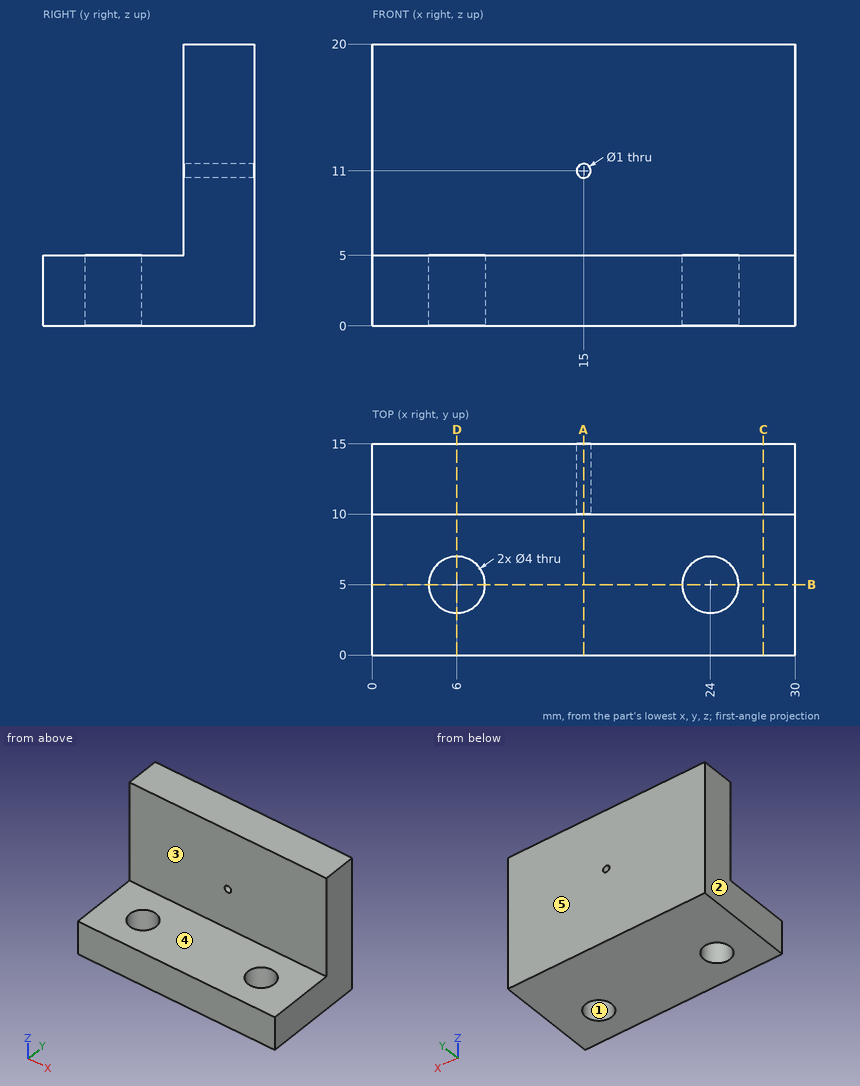
Source: three-view drawing plus pictorial views. Frame: mm from the lowest corner of the part. A direction names the side the tool comes from. Give positions to 0.01 mm unless a question says otherwise; leave off trailing zeros. Write each loop counter-clockwise with the first axis right and the second up, starting at its lowest first coordinate (ties: lowest second). Pieces come first, ordered by that corner, then holes. Notation, with made-up numbers: (-4.5, -3) -> (5.5, -3) arc R29 cw to (5.5, 33) -> close; hole circle Ø3 at (-22.5, 13). An arc over 180 degrees is marked (long way). Write item = value, one per line.
Q1. Cut plane D-D on x = 6. Return loops of the section in (y, z).
Here are the results:
outline = (0, 0) -> (3, 0) -> (3, 5) -> (0, 5) -> close; (7, 0) -> (15, 0) -> (15, 20) -> (10, 20) -> (10, 5) -> (7, 5) -> close
Q2. Cut plane A-A on x = 15. Return loops of the section in (y, z).
Here are the results:
outline = (0, 0) -> (15, 0) -> (15, 10.5) -> (10, 10.5) -> (10, 5) -> (0, 5) -> close; (10, 11.5) -> (15, 11.5) -> (15, 20) -> (10, 20) -> close
Q3. Reachability of the marked faces 4 and 5 from +Z, -Z, +X, -X, +Y, -Y: full face, straight path, thin tool, end or side. Return the list, or none.
Here are the results:
face_4 = +Z, +X, -X, -Y
face_5 = +Z, -Z, +X, -X, +Y
Q4. Cut plane C-C on x = 27.75. Return loops of the section in (y, z).
Here are the results:
outline = (0, 0) -> (15, 0) -> (15, 20) -> (10, 20) -> (10, 5) -> (0, 5) -> close
Q5. Cut plane B-B on y = 5. Return loops of the section in (x, z), then the cut area to 3 significant figures.
Here are the results:
outline = (0, 0) -> (4, 0) -> (4, 5) -> (0, 5) -> close; (8, 0) -> (22, 0) -> (22, 5) -> (8, 5) -> close; (26, 0) -> (30, 0) -> (30, 5) -> (26, 5) -> close
area = 110 mm²
Q6. Mould query, pull axis Y, two halves, no side actions, for the marked faces 1, 2 and 3. Classes: +Y half, -Y half, draft (parallel to the pull), parting line (faces both ways), or undercut.
Here are the results:
face_1 = undercut
face_2 = draft
face_3 = -Y half
Q7. Line query: line 1 (Y direction, x = 6, z = 3.2); line 2 (Z direction, x = 15, y = 13.35); line 3 (X direction, y = 11.8, z = 11). Output: solid intervals per line, ascending. Write a range as from..to.
Here are the results:
line_1 = 0..3, 7..15
line_2 = 0..10.5, 11.5..20
line_3 = 0..14.5, 15.5..30
